Could you check a few things on this drawing? It's one solid part, dimensions in mm from its lowest x, y, z. A direction names the side the tool comes from. Round coordinates to 2 decimals unless told otherwise and drop trailing zeros. Loops run counter-clockwise (first coordinate to the right, second up) from the corner with the lowest first, then second, coordinate; pieces in that order, holes last. Notation, with made-up numbers: M 78,31.25 L 109,31.25 A22 ccw 109,58.25 Z; hole C 87.5,79 d4. An arc over 180 degrees is marked long. Write each question's results on one line, items separated by ' | '. Start each with the question number.
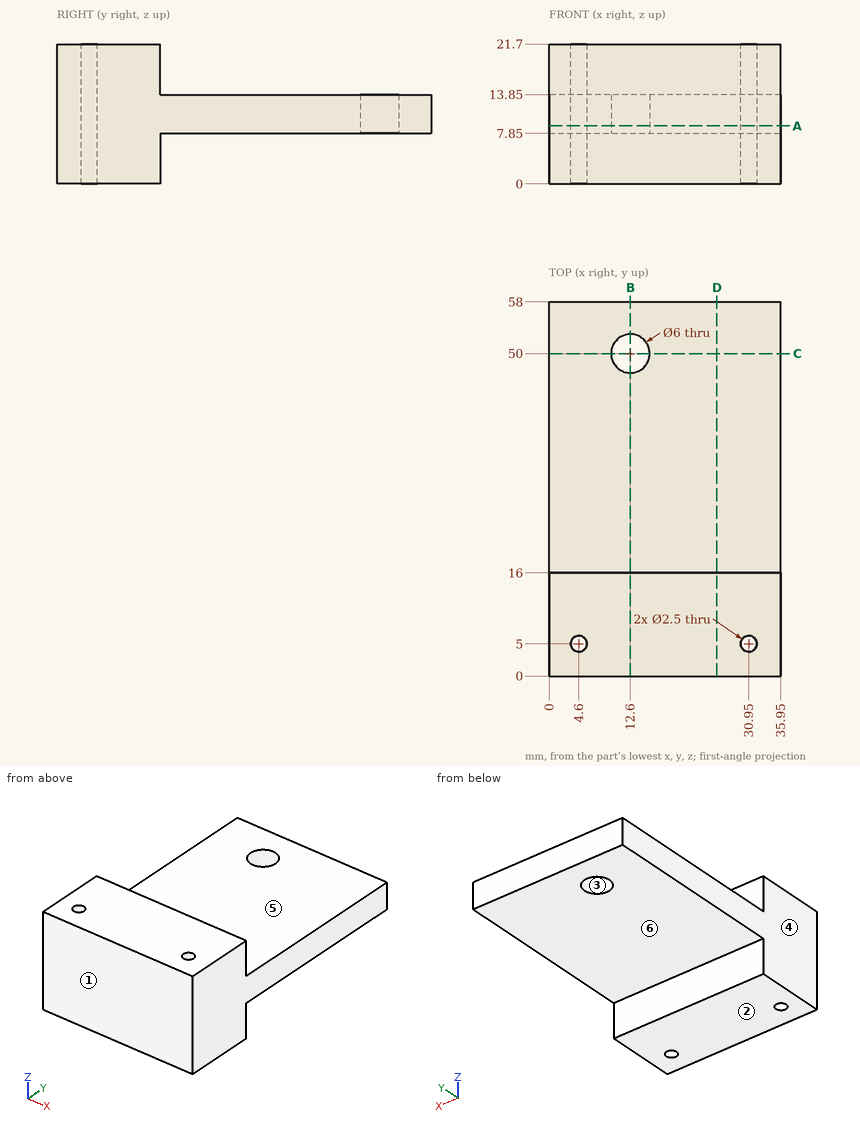
1. I want a section at C-C on y = 50. List the corners of the cut face in (x, z) for me, plus the area to 3 significant figures.
2. Which directions (+Z, -Z, +X, -X, +Y, -Y) give clear straight access to the entire face, cutting with the end or side of a thin tool? Please do the marked faces 4, 5 and 6.
3. I want a section at B-B on x = 12.6. List the corners of the cut face in (y, z) for me.
4. I want a section at A-A on z = 9. List the corners of the cut face in (x, y) for me.
5. I need wall thicknesses on line 1 along X through (y, z) = (5, 15.5); line 2 along X through (y, z) = (50, 10.35); line 3 along Y through (x, z) = (12.6, 12.3). Which ranges of each line are inside material? Lowest first, please.
6. I want a section at D-D on x = 26. List the corners of the cut face in (y, z) for me.
7. For pin 1 (4 mm diameter, centred on x = 13.5, z = 4.5, fed in from +Y); pin 2 (2 mm diameter, centred on x = 29.5, y = 41.5, fed in from -Z), each with a flat end and sliding along its axis, tell me the tip position at first contact or that it passes through.
8. If we mould it in two halves opening along Y, with no side actions, what happens to the marked faces 1, 2 and 3? For each: released by +Y, released by -Y, zero draft, split by the parting line, or undercut.
Outcome:
1) outline: M 0,7.85 L 9.6,7.85 L 9.6,13.85 L 0,13.85 Z; M 15.6,7.85 L 35.95,7.85 L 35.95,13.85 L 15.6,13.85 Z | area: 180 mm2
2) face 4: +Z, -Z, -X, +Y, -Y | face 5: +Z, +X, -X, +Y | face 6: -Z, +X, -X, +Y
3) outline: M 0,0 L 16,0 L 16,7.85 L 47,7.85 L 47,13.85 L 16,13.85 L 16,21.7 L 0,21.7 Z; M 53,7.85 L 58,7.85 L 58,13.85 L 53,13.85 Z
4) outline: M 0,0 L 35.95,0 L 35.95,58 L 0,58 Z; hole C 4.6,5 d2.5; hole C 12.6,50 d6; hole C 30.95,5 d2.5
5) line 1: 0 to 3.35, 5.85 to 29.7, 32.2 to 35.95 | line 2: 0 to 9.6, 15.6 to 35.95 | line 3: 0 to 47, 53 to 58
6) outline: M 0,0 L 16,0 L 16,7.85 L 58,7.85 L 58,13.85 L 16,13.85 L 16,21.7 L 0,21.7 Z
7) pin 1: y = 16 | pin 2: z = 7.85
8) face 1: released by -Y | face 2: zero draft | face 3: undercut
